from build123d import *

# Parameters (mm, degrees)
SKETCH_1_R      = 5
SKETCH_1_R_2    = 1.5
EXTRUDE_1_DEPTH = 3


with BuildPart() as part:
    # 草图1 → 凸台-拉伸1 (new body)
    with BuildSketch(Plane(origin=(0, 0, 0), x_dir=(1, 0, 0), z_dir=(0, 1, 0))):
        with BuildLine():
            Line((135, -2), (135, 24))
            ThreePointArc((135, 24), (133.535533906, 27.535533906), (130, 29))
            Line((130, 29), (119, 29))
            ThreePointArc((119, 29), (115.464466094, 27.535533906), (114, 24))
            Line((114, 24), (114, 22))
            Line((114, 22), (0, 22))
            Line((0, 22), (-80, 22))
            ThreePointArc((-80, 22), (-91, 11), (-80, 0))
            Line((-80, 0), (0, 0))
            Line((0, 0), (114, 0))
            Line((114, 0), (114, -2))
            ThreePointArc((114, -2), (115.464466094, -5.535533906), (119, -7))
            Line((119, -7), (130, -7))
            ThreePointArc((130, -7), (133.535533906, -5.535533906), (135, -2))
        make_face()
        with Locations(Location((-80, 11, 0), (0, 0, 270))):
            Circle(SKETCH_1_R, mode=Mode.SUBTRACT)
        with Locations(Location((124.5, 25.75, 0), (0, 0, 270))):
            Circle(SKETCH_1_R_2, mode=Mode.SUBTRACT)
        with Locations(Location((124.5, -3.75, 0), (0, 0, 270))):
            Circle(SKETCH_1_R_2, mode=Mode.SUBTRACT)
        with Locations(Location((0, 19, 0), (0, 0, 270))):
            Circle(SKETCH_1_R_2, mode=Mode.SUBTRACT)
        with Locations(Location((8, 11, 0), (0, 0, 270))):
            Circle(SKETCH_1_R_2, mode=Mode.SUBTRACT)
        with Locations(Location((0, 3, 0), (0, 0, 270))):
            Circle(SKETCH_1_R_2, mode=Mode.SUBTRACT)
        with Locations(Location((-8, 11, 0), (0, 0, 270))):
            Circle(SKETCH_1_R_2, mode=Mode.SUBTRACT)
    extrude(amount=EXTRUDE_1_DEPTH)


solid = part.part
CAD build for the part. Positions are in the model's coordinates, mm. Give positions to 0.01 mm unless a question says otherwise; leave off trailing zeros. Order: outer loops, then holes, each group sorted by start corner. A loop starts at its lowest first (then second) coordinate and runs counter-clockwise, first axis right, second up. Notation, with made-up numbers: (-23.75, 84) -> (4.25, 84) arc R16 cw to (4.25, 100) -> close; hole circle Ø6 at (-38, 49). An arc over 180 degrees is marked (long way). Return JSON: item names as keys, results as strings.
Q1. Mould opens along Z. For faces 1 (the face through (-84.88, 1.48, -12.08)), 2 (the face through (46, 0, -11)), 3 (the face through (116, 1, -28)) say: pulls with the +Z half, pulls with the -Z half, needs draft (parallel to the pull), parting line crosses it, or undercut.
Working result:
{"face 1": "undercut", "face 2": "needs draft", "face 3": "pulls with the -Z half"}
Q2. Saw through at B-B (x = 89). Write the cut outline in (y, z).
Working result:
{"outline": "(0, -22) -> (3, -22) -> (3, 0) -> (0, 0) -> close"}
Q3. Saw through at A-A (y = 1.55). Write the cut outline in (x, z).
Working result:
{"outline": "(-80, -22) -> (114, -22) -> (114, -24) arc R5 ccw to (119, -29) -> (130, -29) arc R5 ccw to (135, -24) -> (135, 2) arc R5 ccw to (130, 7) -> (119, 7) arc R5 ccw to (114, 2) -> (114, 0) -> (-80, 0) arc R11 ccw to start; hole circle Ø10 at (-80, -11); hole circle Ø3 at (-8, -11); hole circle Ø3 at (0, -19); hole circle Ø3 at (0, -3); hole circle Ø3 at (8, -11); hole circle Ø3 at (124.5, -25.75); hole circle Ø3 at (124.5, 3.75)"}
Q4. Drill centre lines: line 1 (X direction, y = 0.8, z = -11); line 2 (Z direction, x = 124.5, y = 1.9); line 3 (X direction, y = 1, z = -10.5). Where is each one in solid material? Low to high.
Working result:
{"line 1": "-91 to -85, -75 to -9.5, -6.5 to 6.5, 9.5 to 135", "line 2": "-29 to -27.25, -24.25 to 2.25, 5.25 to 7", "line 3": "-90.99 to -84.97, -75.03 to -9.41, -6.59 to 6.59, 9.41 to 135"}
Q5. Flat gauge pins, fed straight in: pin 1 (1.5 mm diameter, centred on x = 29.5, y = 2, fed in from +Z); pin 2 (1.5 mm diameter, centred on y = 1, z = 2, fed in from -X). Where does each tip first touch, or does it go through?
Working result:
{"pin 1": "z = 0", "pin 2": "x = 114"}
